from build123d import *

# Parameters (mm, degrees)
F0_W     = 80
F0_H     = 40
F0_R     = 12.5
F1_DEPTH = 5
F2_W     = 10
F2_H     = 40
F3_DEPTH = 75
F5_DEPTH = 10.001


with BuildPart() as f1:
    # F0 (on Front) → F1 (new body)
    with BuildSketch(Plane.XZ):
        Rectangle(F0_W, F0_H)
        Circle(F0_R, mode=Mode.SUBTRACT)
    extrude(amount=F1_DEPTH)

    # F2 (on face) → F3 (join)
    with BuildSketch(Plane.XZ.offset(5)):
        with Locations((-35, 0)):
            Rectangle(F2_W, F2_H)
    extrude(amount=F3_DEPTH)

    # F4 (on face) → F5 (cut, through all)
    with BuildSketch(Plane.YZ.offset(-30)):
        with BuildLine():
            ThreePointArc((-32.5, 0), (-35.4289321881, 7.0710678119), (-42.5, 10))
            Line((-42.5, 10), (-42.5, -10))
            ThreePointArc((-42.5, -10), (-35.4289321881, -7.0710678119), (-32.5, 0))
        make_face()
        with BuildLine():
            Line((-42.5, -10), (-42.5, 10))
            ThreePointArc((-42.5, 10), (-52.5, 0), (-42.5, -10))
        make_face()
    extrude(amount=-F5_DEPTH, mode=Mode.SUBTRACT)


solid = f1.part
Verification items for the finished model (mm, model axes). A direction names the side the tool comes from. Round coordinates to 2 decimals unless told otherwise and drop trailing zeros. Write each loop counter-clockwise with the first axis right and the second up, starting at its lowest first coordinate (ties: lowest second). Pieces come first, ordered by that corner, then holes.
(1) Section check A-A (x = 0). Enter the section's corners in (y, z).
Returned:
outline: (-5, -20) - (0, -20) - (0, -12.5) - (-5, -12.5) - close; (-5, 12.5) - (0, 12.5) - (0, 20) - (-5, 20) - close
(2) Material ranges on line 1 (Z direction, x = 0, y = -2); line 2 (Y direction, x = -17, z = 9); line 3 (X direction, y = -9, z = -15), recorded low to high.
Returned:
line 1: z = -20 to -12.5, 12.5 to 20
line 2: y = -5 to 0
line 3: x = -40 to -30
(3) Depth check by flat-ended pin: pin 1 Ø1.5 at (y, z) = (-50.5, -9.5) entering from +X; pin 2 Ø12 at (x, z) = (-1, 13) entering from -Y. Enter the tip coordinate at first touch or a pass-through.
Returned:
pin 1: stops at x = -30
pin 2: stops at y = -5
(4) Mould release check, pull along Z, two halves, no side actions. Record for faces 3 (the flat face through (-9, 0, 9)), 4 (the cylindrical face through (11.923, -2.465, 3.755)), 5 (the flat face through (-33, -28, 20)): pulls with the +Z half, pulls with the -Z half, needs draft (parallel to the pull), parting line crosses it, or undercut.
Returned:
face 3: needs draft
face 4: undercut
face 5: pulls with the +Z half
(5) Section check C-C (y = -16.5). Enter the section's corners in (x, z), plus the area to 3 significant figures.
Returned:
outline: (-40, -20) - (-30, -20) - (-30, 20) - (-40, 20) - close
area: 400 mm2
(6) Access from +Z, -Z, +X, -X, +Y, -Y to the whole of each face (thin tool, end or side, straight path). Record for faces 1 (the flat face through (-30, -34, -9)), 2 (the flat face through (-40, -31, 0)).
Returned:
face 1: +Z, -Z, +X, -Y
face 2: +Z, -Z, -X, +Y, -Y
(7) Section check B-B (z = 8). Enter the section's corners in (x, y).
Returned:
outline: (-40, -80) - (-30, -80) - (-30, -48.5) - (-40, -48.5) - close; (-40, -36.5) - (-30, -36.5) - (-30, -5) - (-9.6, -5) - (-9.6, 0) - (-40, 0) - close; (9.6, -5) - (40, -5) - (40, 0) - (9.6, 0) - close
(8) Section check D-D (z = -3.5). Enter the section's corners in (x, y), plus the area to 3 significant figures.
Returned:
outline: (-40, -80) - (-30, -80) - (-30, -51.87) - (-40, -51.87) - close; (-40, -33.13) - (-30, -33.13) - (-30, -5) - (-12, -5) - (-12, 0) - (-40, 0) - close; (12, -5) - (40, -5) - (40, 0) - (12, 0) - close
area: 843 mm2
